The figure shows three views and two pictorial views of one solid part (mm, origin at its lowest corner). Answer the questions. Give positions to 0.01 mm unless a question says otherwise; leave off trailing zeros. Loops run counter-clockwise (first coordinate to the right, second up) from the corner with the lowest first, then second, coordinate; pieces in that order, holes last. Notation, with made-up numbers: M 28.5,77.5 L 33.5,77.5 A20 cw 33.5,92.5 Z; hole C -31,52.5 d2. An arc over 180 degrees is marked long. One line per item, written item: value. Start each with the question number.
Q1. The mould has two halves that part along X. Classify the marked faces 1, 2 and 3: +X half, -X half, draft (parallel to the pull), parting line (faces both ways), or undercut.
Q2. A cutting plane is placed at B-B, the plane x = 67.5. Determine the outline of the cut face in (y, z).
Q3. Consider L1, parallel to Y at x = 75.25, z = 2.05 (3 decimals); L2, parallel to Y at x = 59.75, z = 1 (3 decimals); L3, parallel to Y at x = 83, z = 2. Determine where each line is inside the solid, lowest interval first.
Q4. Flat-ended cylindrical pins translate along their axes: pin 1 (1.1 mm diameter, centred on x = 59.75, y = 3, fed in from +Z); pin 2 (0.5 mm diameter, centred on x = 61.5, y = 5.5, fed in from +Z). Find the tip coordinate at first contact, or state that the pin passes through.
Q5. A cutting plane is placed at C-C, the plane y = 1.25. Determine the outline of the cut face in (x, z).
Q6. A cutting plane is placed at A-A, the plane z = 1.95. State how many separate pieces and enclosed holes the cut face has, and give its area (3 significant figures).
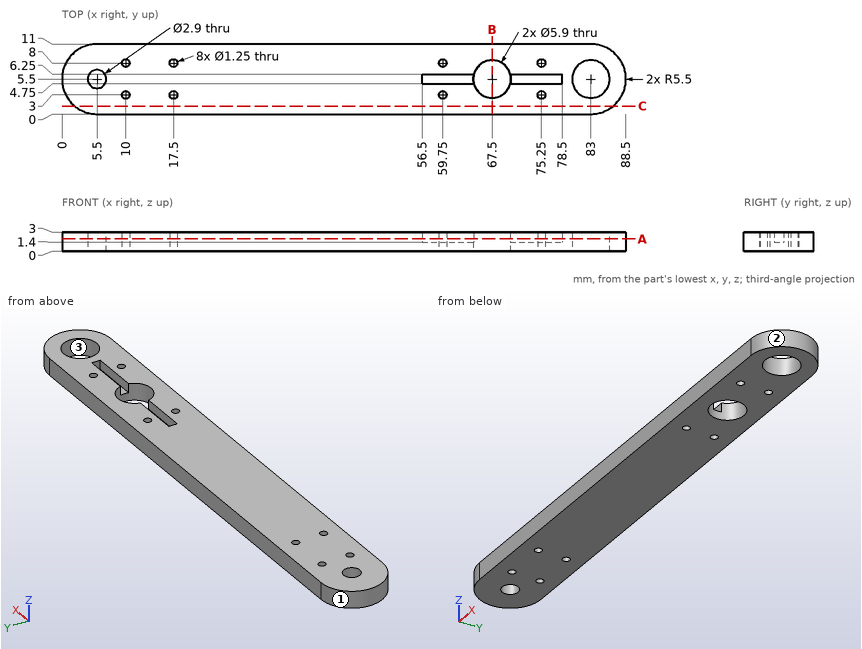
Answer block:
1. face 1: -X half
1. face 2: +X half
1. face 3: undercut
2. outline: M 0,0 L 2.55,0 L 2.55,3 L 0,3 Z; M 8.45,0 L 11,0 L 11,3 L 8.45,3 Z
3. L1: 0 to 2.375, 3.625 to 4.75, 6.25 to 7.375, 8.625 to 11
3. L2: 0 to 2.375, 3.625 to 7.375, 8.625 to 11
3. L3: 0 to 2.55, 8.45 to 11
4. pin 1: through
4. pin 2: z = 1.4
5. outline: M 2.01,0 L 86.49,0 L 86.49,3 L 2.01,3 Z
6. separate pieces: 1
6. enclosed holes: 11
6. area: 852 mm^2
